Geometry: see drawing. Coordinates: mm, zero at the bounding-box minimum. A direction names the side the tool comes from. Coordinates: 2 decimals unless noted, no trailing zeros. Loops run counter-clockwise (first coordinate to the right, second up) from the corner with the lowest first, then second, coordinate; pieces in that order, holes last. Notation, with made-up numbers: (-15.75, 32) - (14.25, 32) arc R16 cw to (14.25, 62) - close; hole circle Ø7 at (-32, 8.5). An arc over 180 degrees is marked (long way). Answer in a Markdown table with one row per item.
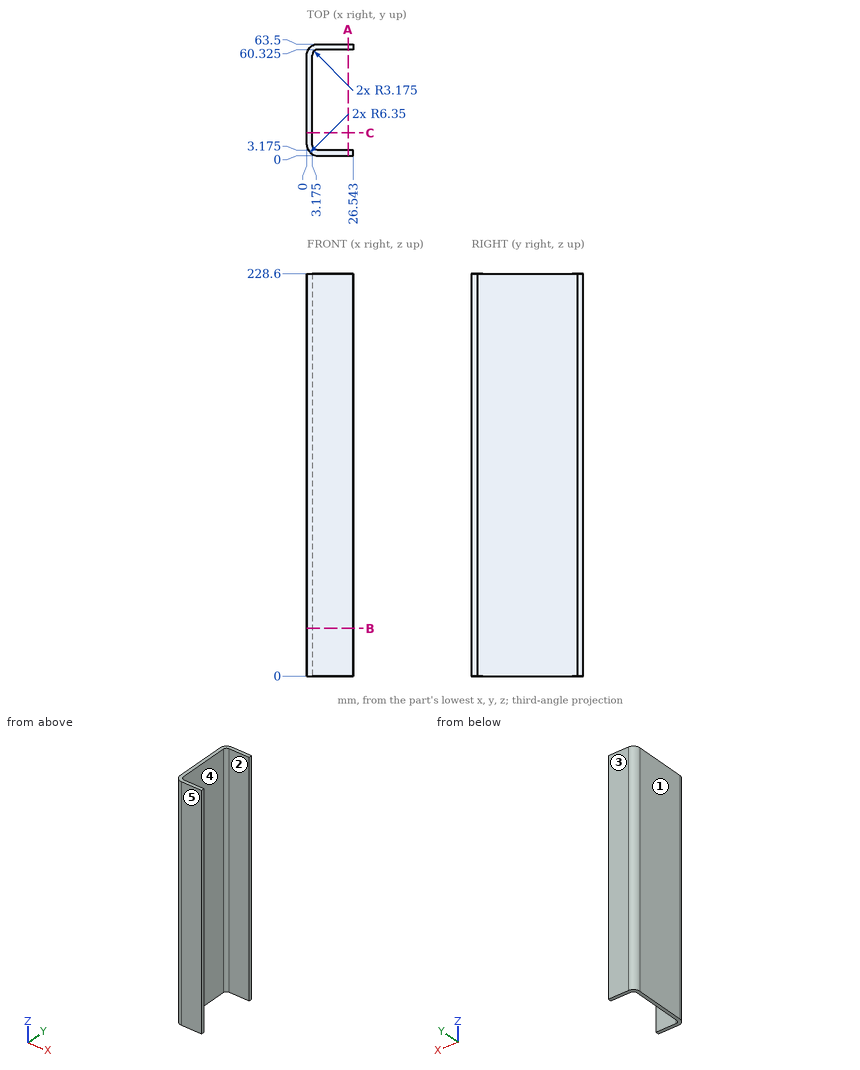
(1) Cut plane C-C on y = 13. Output: boundary loops of the cut face in (x, z) (3 decimals).
Verdict:
| item | result |
|---|---|
| outline | (0, 0) - (3.175, 0) - (3.175, 228.6) - (0, 228.6) - close |
(2) Ray query, probe 1 along Y at (x, z) = (21.5, 145) (3 decimals); probe 2 along X at (y, z) = (15, 36) (3 decimals); probe 3 along Y at (x, z) = (1.75, 83.5). Return the intervals inside material, ascending.
Verdict:
| item | result |
|---|---|
| probe 1 | y = 0 to 3.175, 60.325 to 63.5 |
| probe 2 | x = 0 to 3.175 |
| probe 3 | y = 1.97 to 61.53 |
(3) Access query for the marked faces 1 and 2. Directions: +Z, -Z, +X, -X, +Y, -Y. A direction counts if a zero-diameter tool reaches every point of the face in a straight line with its end or side. Return the directions, or none.
Verdict:
| item | result |
|---|---|
| face 1 | +Z, -Z, -X, +Y, -Y |
| face 2 | +Z, -Z, +X |
(4) Cut plane B-B on z = 27. Output: boundary loops of the cut face in (x, y) (3 decimals).
Verdict:
| item | result |
|---|---|
| outline | (0, 6.35) arc R6.35 ccw to (6.35, 0) - (26.543, 0) - (26.543, 3.175) - (6.35, 3.175) arc R3.175 cw to (3.175, 6.35) - (3.175, 57.15) arc R3.175 cw to (6.35, 60.325) - (26.543, 60.325) - (26.543, 63.5) - (6.35, 63.5) arc R6.35 ccw to (0, 57.15) - close |
(5) Cut plane A-A on x = 23.5. Output: boundary loops of the cut face in (y, z) (3 decimals), then the cut area to 3 significant figures.
Verdict:
| item | result |
|---|---|
| outline | (0, 0) - (3.175, 0) - (3.175, 228.6) - (0, 228.6) - close; (60.325, 0) - (63.5, 0) - (63.5, 228.6) - (60.325, 228.6) - close |
| area | 1,450 mm² |
(6) First-contact query: pin 1 Ø4 at (x, y) = (6.5, 12) entering from -Z; pin 2 Ø10 at (y, z) = (46.5, 155.5) entering from +X (3 decimals); pin 3 Ø4 at (x, z) = (3, 72) entering from -Y. Flat tips, straight axial feed; report the tip coordinate or a pass-through.
Verdict:
| item | result |
|---|---|
| pin 1 | passes through |
| pin 2 | stops at x = 3.175 |
| pin 3 | stops at y = 0.15 |
(7) Pull-direction query (Y, two-part tool) for the marked faces 3, 4 and 5; classes: pulls with the +Y half, pulls with the -Y half, needs draft (parallel to the pull), parting line crosses it, or undercut.
Verdict:
| item | result |
|---|---|
| face 3 | pulls with the +Y half |
| face 4 | undercut |
| face 5 | pulls with the -Y half |
